Autodesk Inventor part; units mm, degrees
ref_plane "YZ Plane" through (0, 0, 0) normal (1, 0, 0) x (0, 1, 0)
ref_plane "XZ Plane" through (0, 0, 0) normal (0, 1, 0) x (-1, 0, 0)
ref_plane "XY Plane" through (0, 0, 0) normal (0, 0, 1) x (1, 0, 0)
sketch "Sketch1" plane through (0, 0, 0) normal (0, 1, 0) x (-1, 0, 0)
  line L0 (4.7584, -0.779) -> (21.7584, -0.779)
  line L1 (21.7584, -0.779) -> (21.7584, -13.779)
  line L2 (21.7584, -13.779) -> (4.7584, -13.779)
  line L3 (4.7584, -13.779) -> (4.7584, -0.779)
  line L4 (8.7584, -3.779) -> (17.7584, -3.779)
  line L5 (17.7584, -3.779) -> (17.7584, -9.779)
  line L6 (17.7584, -9.779) -> (8.7584, -9.779)
  line L7 (8.7584, -9.779) -> (8.7584, -3.779)
  line L8 (21.7584, -0.779) -> (-18.2416, -0.779)
  line L9 (-18.2416, -0.779) -> (-18.2416, 5.221)
  line L10 (-18.2416, 5.221) -> (21.7584, 5.221)
  line L11 (21.7584, 5.221) -> (21.7584, -0.779)
  line L12 (17.7584, -6.6245) -> (21.7584, -6.6245) construction
  line L13 (8.7584, -6.779) -> (4.7584, -6.779) construction
  line L14 (-18.2416, -0.779) -> (-1.2416, -0.779)
  line L15 (-1.2416, -0.779) -> (-1.2416, -13.779)
  line L16 (-1.2416, -13.779) -> (-18.2416, -13.779)
  line L17 (-18.2416, -13.779) -> (-18.2416, -0.779)
  line L18 (-14.2416, -3.779) -> (-5.2416, -3.779)
  line L19 (-5.2416, -3.779) -> (-5.2416, -9.779)
  line L20 (-5.2416, -9.779) -> (-14.2416, -9.779)
  line L21 (-14.2416, -9.779) -> (-14.2416, -3.779)
  line L22 (-5.2416, -6.779) -> (-1.2416, -6.779) construction
  line L23 (-18.2416, -6.779) -> (-14.2416, -6.779) construction
  line L24 (21.7584, 5.221) -> (4.7584, 5.221)
  line L25 (4.7584, 5.221) -> (4.7584, 15.221)
  line L26 (4.7584, 15.221) -> (21.7584, 15.221)
  line L27 (21.7584, 15.221) -> (21.7584, 5.221)
  line L28 (-18.2416, 5.221) -> (-1.2416, 5.221)
  line L29 (-1.2416, 5.221) -> (-1.2416, 15.221)
  line L30 (-1.2416, 15.221) -> (-18.2416, 15.221)
  line L31 (-18.2416, 15.221) -> (-18.2416, 5.221)
  point P0 (0, 0)
  dimension "d0" = 9
  dimension "d1" = 6
  dimension "d2" = 4
  dimension "d3" = 40
  dimension "d4" = 6
  dimension "d5" = 4
  dimension "d6" = 3
  dimension "d7" = 4
  dimension "d8" = 9
  dimension "d9" = 6
  dimension "d10" = 3
  dimension "d11" = 4
  dimension "d14" = 10
  dimension "d15" = 10
extrude "Extrusion1" add sketch "Sketch1" along normal blind 6
equation "\"d5\" = d2"
equation "\"d7\" = d2"
equation "\"d8\" = d0"
equation "\"d9\" = d1"
equation "\"d10\" = d6"
equation "\"d11\" = d5"
equation "\"d15\" = d14"
properties part number "flipper-holder"
Build history of the part. All positions in model axes, mm. A direction names the side the tool comes from. Round coordinates to 2 decimals unless told otherwise and drop trailing zeros. Order: outer loops, then holes, each group sorted by start corner. A loop starts at its lowest first (then second) coordinate and runs counter-clockwise, first axis right, second up. Notation, with made-up numbers: (-30.75, 17) - (19.25, 17) arc R21 ccw to (19.25, 49) - close; hole circle Ø5 at (37, 54). An arc over 180 degrees is marked (long way). Use a Markdown table: item, result.
1) Saw through at C-C on y = 2.5. Write the cut outline in (x, z).
Recorded:
| item | result |
|---|---|
| outline | (-21.76, -13.78) - (-4.76, -13.78) - (-4.76, -0.78) - (1.24, -0.78) - (1.24, -13.78) - (18.24, -13.78) - (18.24, 15.22) - (1.24, 15.22) - (1.24, 5.22) - (-4.76, 5.22) - (-4.76, 15.22) - (-21.76, 15.22) - close; hole (-17.76, -9.78) - (-8.76, -9.78) - (-8.76, -3.78) - (-17.76, -3.78) - close; hole (5.24, -9.78) - (14.24, -9.78) - (14.24, -3.78) - (5.24, -3.78) - close |
2) Saw through at A-A on z = -8.5. Write the cut outline in (x, y), and give its area (3 significant figures).
Recorded:
| item | result |
|---|---|
| outline | (-21.76, 0) - (-17.76, 0) - (-17.76, 6) - (-21.76, 6) - close; (-8.76, 0) - (-4.76, 0) - (-4.76, 6) - (-8.76, 6) - close; (1.24, 0) - (5.24, 0) - (5.24, 6) - (1.24, 6) - close; (14.24, 0) - (18.24, 0) - (18.24, 6) - (14.24, 6) - close |
| area | 96.0 mm² |
3) Wall check: L1, parallel to X at y = 2.2, z = -5; L2, parallel to Z at x = 9.5, y = 3.8; L3, parallel to X at y = 5.2, z = -2.25. Give the ranges that are in metal, low to high.
Recorded:
| item | result |
|---|---|
| L1 | x = -21.76 to -17.76, -8.76 to -4.76, 1.24 to 5.24, 14.24 to 18.24 |
| L2 | z = -13.78 to -9.78, -3.78 to 15.22 |
| L3 | x = -21.76 to -4.76, 1.24 to 18.24 |
4) Saw through at D-D on z = 10. Write the cut outline in (x, y).
Recorded:
| item | result |
|---|---|
| outline | (-21.76, 0) - (-4.76, 0) - (-4.76, 6) - (-21.76, 6) - close; (1.24, 0) - (18.24, 0) - (18.24, 6) - (1.24, 6) - close |
5) Tool access for faces 4 (the face through (-2, 3, 5.221)), 5 (the face through (-8.758, 3, -7)), 6 (the face through (10, 3, 15.221)), 7 (the face through (-4.758, 3, -7)): list every direction of +Z, -Z, +X, -X, +Y, -Y with a clear straight run to the whole face (end or side of a thin tool).
Recorded:
| item | result |
|---|---|
| face 4 | +Z, +Y, -Y |
| face 5 | +Y, -Y |
| face 6 | +Z, +X, -X, +Y, -Y |
| face 7 | -Z, +Y, -Y |
6) Pull direction Z, two halves, no side cores. Call faces 1 (the face through (-2, 3, -0.779)), 2 (the face through (-13, 3, -9.779)), 3 (the face through (1.242, 3, -7)): pulls with the +Z half, pulls with the -Z half, needs draft (parallel to the pull), parting line crosses it, or undercut.
Recorded:
| item | result |
|---|---|
| face 1 | pulls with the -Z half |
| face 2 | undercut |
| face 3 | needs draft |
7) Saw through at B-B on x = -16.5. Write the cut outline in (y, z).
Recorded:
| item | result |
|---|---|
| outline | (0, -13.78) - (6, -13.78) - (6, -9.78) - (0, -9.78) - close; (0, -3.78) - (6, -3.78) - (6, 15.22) - (0, 15.22) - close |
